```python
from build123d import *

# Parameters (mm, degrees)
SKETCH4_R = 0.508


with BuildPart() as part:
    # Sweep1: sweep along a curve in space
    with BuildLine() as sweep1_path:
        Line((15.748, 6.604, -4.969858904), (15.748, 1.27, -4.969858904))
        ThreePointArc((15.748, 1.27, -4.969858904), (15.413671635, 0.371974388, -5.132921743), (14.606531561, 0, -5.52659026))
        Line((14.606531561, 0, -5.52659026), (5.97077017, 0, -9.738532518))
        ThreePointArc((5.97077017, 0, -9.738532518), (4.519904893, 0, -9.865466782), (3.356766269, 0, -8.988978961))
        Line((3.356766269, 0, -8.988978961), (0.971149403, 0, -5.171193917))
        ThreePointArc((0.971149403, 0, -5.171193917), (0.890159133, 0, -2.078300277), (3.556, 0, -0.508))
        Line((3.556, 0, -0.508), (16.463402457, 0, -0.508))
        ThreePointArc((16.463402457, 0, -0.508), (17.321402021, 0, -0.841657782), (17.728569724, 0, -1.667312207))
        Line((17.728569724, 0, -1.667312207), (18.289933093, 0, -8.083724883))
    # Sketch4 → Sweep1 (sweep)
    with BuildSketch(Plane(origin=(0, 6.604, 0), x_dir=(1, 0, 0), z_dir=(0, 1, 0))):
        with Locations((15.748, 4.969858904)):
            Circle(SKETCH4_R)
    sweep(path=sweep1_path.line)


solid = part.part
```
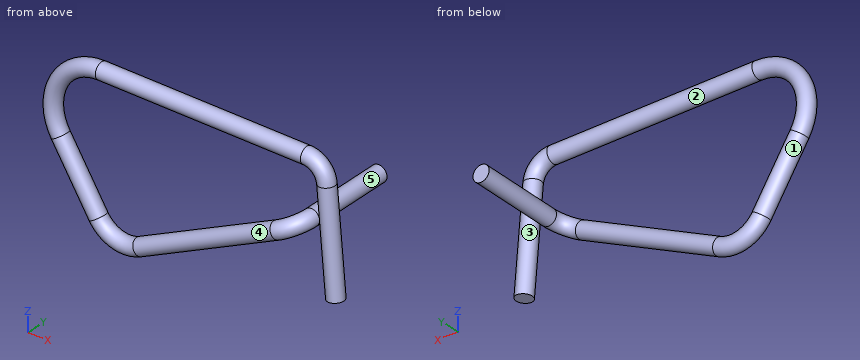
For this review, take the finished solid that the model builds, in its own axes (mm). Face numbers are marked on the shaded views. A direction names the side the tool comes from. Give positions to 0.01 mm unless a question says otherwise; leave off trailing zeros. Order: outer loops, then holes, each group sorted by start corner. A loop starts at its lowest first (then second) coordinate and runs counter-clockwise, first axis right, second up.
1) Insertion check: pin 1 (1 mm diameter, centred on x = 3.5, z = -9, fed in from +Y); pin 2 (3 mm diameter, centred on y = 1.5, z = -2, fed in from +X); pin 3 (5 mm diameter, centred on x = 13.5, z = -3.5, fed in from +Y); pin 4 (3 mm diameter, centred on y = 6, z = -3.5, fed in from -X). Each pin has a flat end and moves straight along its axis. Give the tip position at first contact, or say it passes through.
2) Wall thickness on line 1 (X direction, y = 0.25, z = -3.25); line 2 (X direction, y = 2.5, z = -5); line 3 (Y direction, x = 1.25, z = -4.75): over which ranges is each line inside the solid? List them lowest first.
3) For the marked faces 4 and 5, list the 3-axis set-ups (+Z, -Z, +X, -X, +Y, -Y) from which the entire face can be reached by the end or side of a thin tool; tool diameter is ignored.
4) Take a section at A-A (y = 6). Give the boundary of the cut face in (x, z).
5) The part is to be moulded in two halves that separate along Z. For the marked faces 1, 2 and 3, say which applies: released by +Z, released by -Z, zero draft, split by the parting line, or undercut.
Derived:
1. pin 1: stops at y = 0.51
1. pin 2: stops at x = 18.3
1. pin 3: stops at y = 6.6
1. pin 4: stops at x = 15.24
2. line 1: x = 0.08 to 0.97, 17.42 to 18.31
2. line 2: x = 15.24 to 16.26
2. line 3: y = -0.23 to 0.23
3. face 4: none
3. face 5: +Y
4. outline: circle Ø1.02 at (15.75, -4.97)
5. face 1: undercut
5. face 2: undercut
5. face 3: split by the parting line
